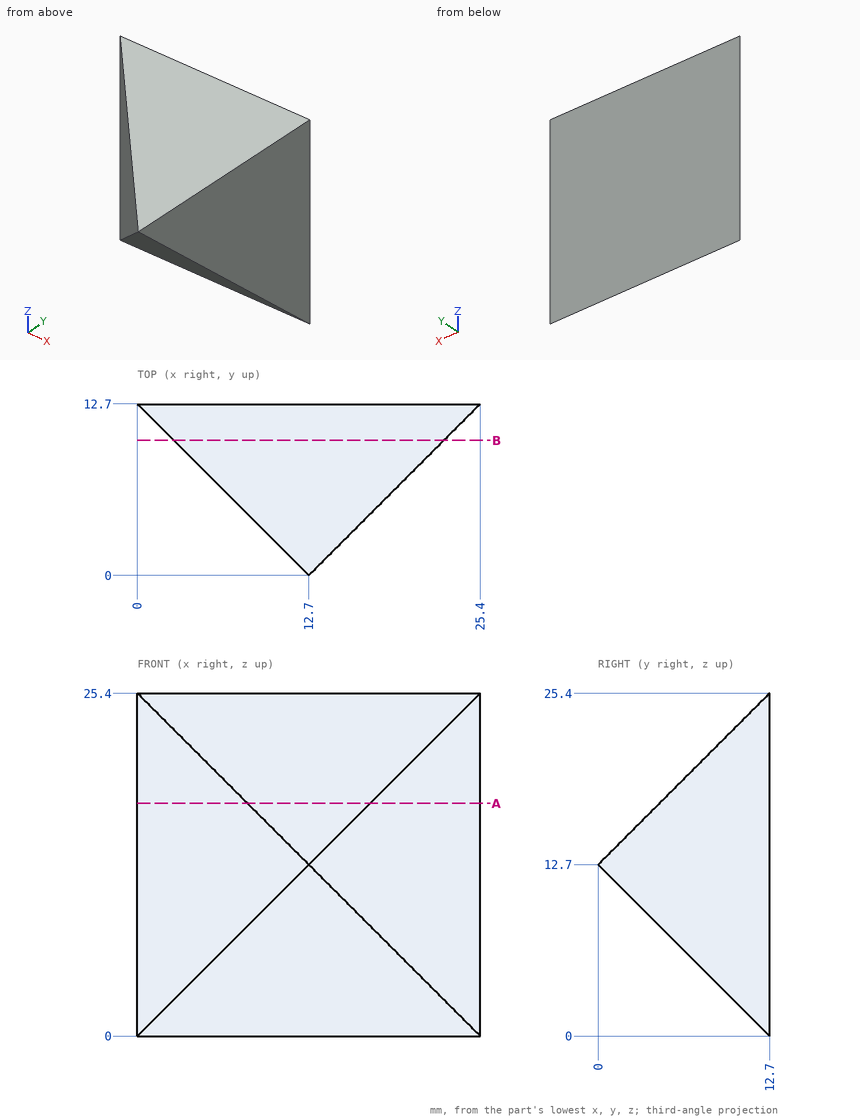
Source: three-view drawing plus pictorial views. Frame: mm from the lowest corner of the part. Round coordinates to 2 decimals unless told otherwise and drop trailing zeros. Loops run counter-clockwise (first coordinate to the right, second up) from the corner with the lowest first, then second, coordinate; pieces in that order, holes last. Notation, with made-up numbers: (-6.75, -31.5) - (20.25, -31.5) arc R21 ccw to (20.25, -7.5) - close; hole circle Ø10 at (47, -20.5). An arc over 180 degrees is marked (long way). Write item = value, one per line. Start each with the question number.
Item 1: First-contact query: pin 1 Ø5 at (x, y) = (19, 11) entering from +Z; pin 2 Ø6 at (y, z) = (10.5, 8) entering from -X; pin 3 Ø8 at (x, z) = (16.5, 13) entering from -Y; pin 4 Ø6 at (x, z) = (6, 19) entering from -Y. Flat tips, straight axial feed; report the tip coordinate or a pass-through.
Item 2: Section query A-A on z = 17.25. Output: boundary loops of the cut face in (x, y), plus the area to 3 significant figures.
Item 3: Material intervals for line 1 (X direction, y = 3.75, z = 15); line 2 (Y direction, x = 20, z = 12.5); line 3 (Z direction, x = 12, y = 5.25), sorted ascending.
Item 4: Section query B-B on y = 10. Output: boundary loops of the cut face in (x, z).
Results list:
q1.pin_1 = 25.4
q1.pin_2 = 0
q1.pin_3 = 0
q1.pin_4 = 4.39
q2.outline = (0, 12.7) - (8.15, 4.55) - (17.25, 4.55) - (25.4, 12.7) - close
q2.area = 141 mm²
q3.line_1 = 8.95 to 16.45
q3.line_2 = 7.3 to 12.7
q3.line_3 = 7.45 to 17.95
q4.outline = (2.7, 2.7) - (22.7, 2.7) - (22.7, 22.7) - (2.7, 22.7) - close
